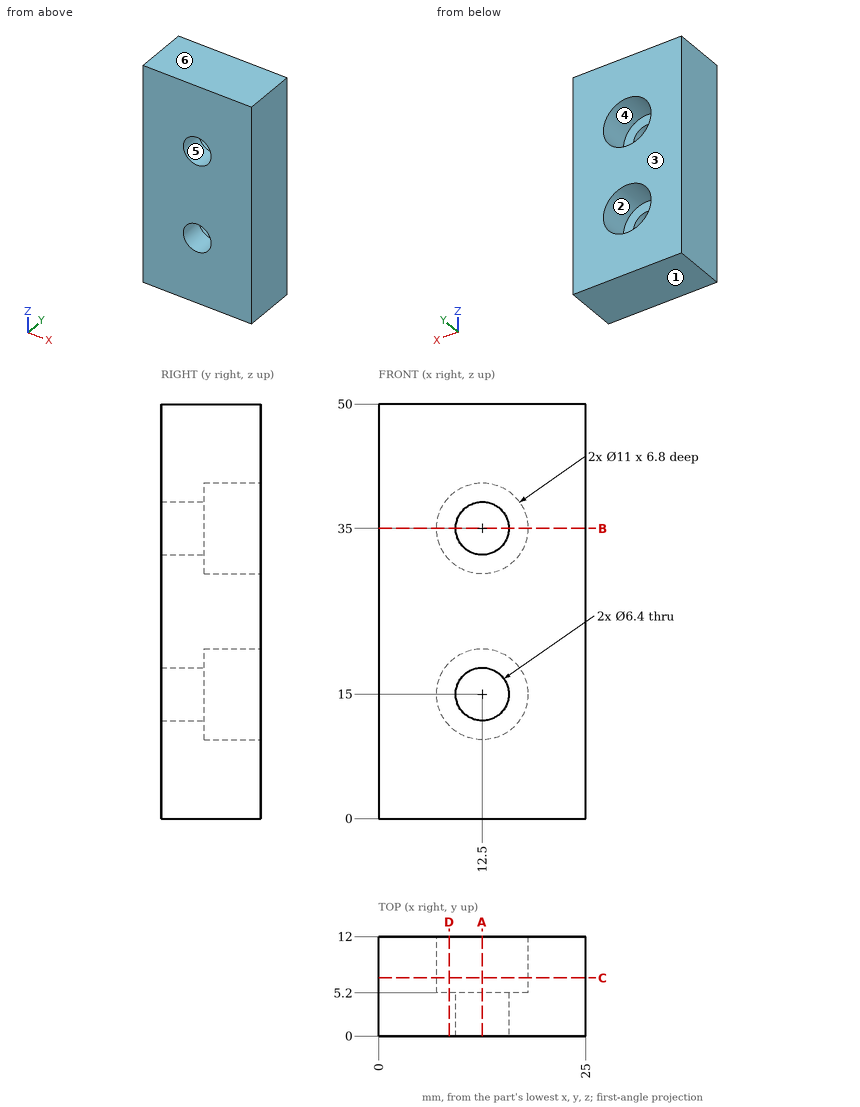
For this review, use the dimensioned drawing (mm, ordinates from the lowest corner) and the shaded views. A direction names the side the tool comes from. Round coordinates to 2 decimals unless told otherwise and drop trailing zeros. Write each loop counter-clockwise with the first axis right and the second up, starting at its lowest first coordinate (ties: lowest second). Pieces come first, ordered by that corner, then holes. Notation, with made-up numbers: M 20,10 L 45,10 A28 cw 45,36 Z; hole C 84,74.5 d10. An arc over 180 degrees is marked long. Write item = value, one per line. Start each with the question number.
(1) We need section A-A (x = 12.5). Give the boundary of the cut face in (y, z), then the cut area to 3 significant figures.
(2) We need section D-D (x = 8.5). Give the boundary of the cut face in (y, z).
(3) For line 1 along Z through (x, y) = (12.5, 8.5); line 2 along Z through (x, y) = (12.5, 2.05); line 3 along X through (y, z) = (4.1, 15), list the stretches that pass through material, from the lowest coordinate up.
(4) Clearance check with flat-ended pins moving along their axes: pin 1 Ø1.5 at (x, y) = (14.5, 3.5) entering from -Z; pin 2 Ø3.5 at (x, z) = (12, 37) entering from +Y; pin 3 Ø4 at (x, z) = (12.5, 35) entering from +Y. State where each tip first meets the part, or that it passes through.
(5) For the marked faces 1 and 2, list the 3-axis set-ups (+Z, -Z, +X, -X, +Y, -Y) from which the entire face can be reached by the end or side of a thin tool; tool diameter is ignored.
(6) We need section B-B (z = 35). Give the boundary of the cut face in (x, y), then the cut area to 3 significant figures.
(7) We need section C-C (y = 7). Give the boundary of the cut face in (x, z), then the cut area to 3 significant figures.
(8) The part is to be moulded in two halves that separate along Z. For the marked faces 3, 4, 5 and 6, say which applies: +Z half, -Z half, draft (parallel to the pull), parting line (faces both ways), or undercut.
Results found:
q1.outline = M 0,0 L 12,0 L 12,9.5 L 5.2,9.5 L 5.2,11.8 L 0,11.8 Z; M 0,18.2 L 5.2,18.2 L 5.2,20.5 L 12,20.5 L 12,29.5 L 5.2,29.5 L 5.2,31.8 L 0,31.8 Z; M 0,38.2 L 5.2,38.2 L 5.2,40.5 L 12,40.5 L 12,50 L 0,50 Z
q1.area = 384 mm²
q2.outline = M 0,0 L 12,0 L 12,11.23 L 5.2,11.23 L 5.2,18.77 L 12,18.77 L 12,31.23 L 5.2,31.23 L 5.2,38.77 L 12,38.77 L 12,50 L 0,50 Z
q3.line_1 = 0 to 9.5, 20.5 to 29.5, 40.5 to 50
q3.line_2 = 0 to 11.8, 18.2 to 31.8, 38.2 to 50
q3.line_3 = 0 to 9.3, 15.7 to 25
q4.pin_1 = 0
q4.pin_2 = 5.2
q4.pin_3 = through
q5.face_1 = -Z, +X, -X, +Y, -Y
q5.face_2 = +Y
q6.outline = M 0,0 L 9.3,0 L 9.3,5.2 L 7,5.2 L 7,12 L 0,12 Z; M 15.7,0 L 25,0 L 25,12 L 18,12 L 18,5.2 L 15.7,5.2 Z
q6.area = 192 mm²
q7.outline = M 0,0 L 25,0 L 25,50 L 0,50 Z; hole C 12.5,15 d11; hole C 12.5,35 d11
q7.area = 1,060 mm²
q8.face_3 = draft
q8.face_4 = undercut
q8.face_5 = undercut
q8.face_6 = +Z half
